The model under review builds one solid part; all positions refer to its coordinate system, in mm. A direction names the side the tool comes from. Round coordinates to 2 decimals unless told otherwise and drop trailing zeros. Loops run counter-clockwise (first coordinate to the right, second up) from the corner with the lowest first, then second, coordinate; pieces in that order, holes last. Notation, with made-up numbers: (60.5, -7.75) - (112.5, -7.75) arc R31 ccw to (112.5, 26.25) - close; hole circle Ø11 at (40.5, 13.5). An arc over 180 degrees is marked (long way). Answer as CSV lines item,"result".
from build123d import *

# Parameters (mm, degrees)
F2_R = 0.5


with BuildPart() as f1:
    # F0 (on Right) → F1 (revolve)
    with BuildSketch(Plane.YZ):
        Polygon((0, 100), (0, 0), (319.253526, 0), (319.253526, 50.35), (308.253526, 50.35), (308.253526, 48.35), (304.253526, 48.35), (304.253526, 58), (14.253526, 58), (14.253526, 87.1), (18.253526, 87.1), (18.253526, 85.1), (34.253526, 85.1), (34.253526, 100), align=None)
    revolve(axis=Axis((0, 159.626763, 0), (0, 1, 0)))

    # F2
    f2_edges = [f1.edges().sort_by_distance(p)[0] for p in [
        (0, 319.253526, -50.35),
        (0, 304.253526, -48.35),
        (0, 304.253526, -58),
        (0, 34.253526, -85.1),
        (0, 34.253526, -100),
    ]]
    fillet(f2_edges, radius=F2_R)


solid = f1.part
1. Draft analysis for pull direction Y (two halves, no side actions). For faces 1 (the face through (32.677, 306.479, -35.636)), 2 (the face through (74, 34.254, -44)), 3 (the face through (-51.46, 156.98, 26.76)), state which applies: +Y half, -Y half, draft (parallel to the pull), parting line (faces both ways), or undercut.
Numbers:
face 1,"undercut"
face 2,"+Y half"
face 3,"draft"
2. Wall thickness on probe 1 along X at (y, z) = (25, 0); probe 2 along X at (y, z) = (16.65, 0); probe 3 along Y at (x, z) = (34.5, -45): over which ranges is each line inside the solid? List them lowest first.
Numbers:
probe 1,"x = -100 to -85.1, -58 to 58, 85.1 to 100"
probe 2,"x = -100 to -87.1, -58 to 58, 87.1 to 100"
probe 3,"y = 0 to 304.25"
3. Tool access review of faces 4 (the face through (-30.637, 313.43, -39.956)), 5 (the face through (-18.9, 18.254, 83.5)), 6 (the face through (1, 0, -1)): name each direction out of +Z, -Z, +X, -X, +Y, -Y from which nothing blocks a thin tool from reaching the whole face with its end or side.
Numbers:
face 4,"+Y"
face 5,"none"
face 6,"+Z, -Z, +X, -X, -Y"
4. Take a section at C-C (y = 283.5). State the section outline as (x, z) points, plus the area to 3 significant figures.
Numbers:
outline,"circle Ø116 at (0, 0)"
area,"10,600 mm²"
5. Clearance check with flat-ended pins moving along their axes: pin 1 (6 mm diameter, centred on x = 56.5, y = 265.5, fed in from +Z); pin 2 (10 mm diameter, centred on x = -49.5, y = 218.5, fed in from -Z); pin 3 (2 mm diameter, centred on x = 70, z = -15.5, fed in from +Y). State where each tip first meets the part, or that it passes through.
Numbers:
pin 1,"stops at z = 22.4"
pin 2,"stops at z = -37.2"
pin 3,"stops at y = 14.25"
